from build123d import *

# Parameters (mm, degrees)
SKETCH_1_W             = 60
SKETCH_1_H             = 60
SKETCH_1_R             = 17.5
EXTRUDE_1_DEPTH        = 80
HOLE_WIZARD_M6_1_D     = 5
HOLE_WIZARD_M6_1_DEPTH = 17
HOLE_WIZARD_M6_1_TIP   = 1.502151548


with BuildPart() as part:
    # Sketch 1 → Extrude 1 (new body)
    with BuildSketch(Plane(origin=(0, 0, 0), x_dir=(0, 0, -1), z_dir=(1, 0, 0))):
        Rectangle(SKETCH_1_W, SKETCH_1_H)
        Circle(SKETCH_1_R, mode=Mode.SUBTRACT)
    extrude(amount=EXTRUDE_1_DEPTH)

    # Sketch 6 → Cut-Revolve 5 (revolve, cut)
    with BuildSketch(Plane.XY, mode=Mode.PRIVATE) as cut_revolve_5_sk:
        Polygon((0, 17.5), (2.5, 17.5), (2.5, 20.547619048), (2, 20.547619048), (2, 22.833333333), (0, 22.833333333), align=None)
    revolve(cut_revolve_5_sk.sketch.rotate(Axis((80, 0, 0), (-1, 0, 0)), 270), axis=Axis((80, 0, 0), (-1, 0, 0)), mode=Mode.SUBTRACT)

    # Sketch 7 → Cut-Revolve 6 (revolve, cut)
    with BuildSketch(Plane.XY, mode=Mode.PRIVATE) as cut_revolve_6_sk:
        Polygon((77.5, 17.5), (80, 17.5), (80, 22.833333333), (78, 22.833333333), (78, 20.547619048), (77.5, 20.547619048), align=None)
    revolve(cut_revolve_6_sk.sketch.rotate(Axis((80, 0, 0), (-1, 0, 0)), 270), axis=Axis((80, 0, 0), (-1, 0, 0)), mode=Mode.SUBTRACT)

    # Hole Wizard M6 _1
    with Locations(Plane.XY.offset(30)):
        with Locations((15, 20), (15, -20), (65, -20), (65, 20)):
            Hole(HOLE_WIZARD_M6_1_D / 2, depth=HOLE_WIZARD_M6_1_DEPTH)
            with Locations((0, 0, -(HOLE_WIZARD_M6_1_DEPTH + HOLE_WIZARD_M6_1_TIP / 2))):  # 118° drill point
                Cone(0, HOLE_WIZARD_M6_1_D / 2, HOLE_WIZARD_M6_1_TIP, mode=Mode.SUBTRACT)


solid = part.part
Can you work these out from the model? Positions are in its coordinate system, mm. A direction names the side the tool comes from. Give positions to 0.01 mm unless a question says otherwise; leave off trailing zeros. Order: outer loops, then holes, each group sorted by start corner. A loop starts at its lowest first (then second) coordinate and runs counter-clockwise, first axis right, second up. Notation, with made-up numbers: M -3.75,17.5 L 55.25,17.5 A18 cw 55.25,36.5 Z; hole C 30.25,69 d11. An arc over 180 degrees is marked long. Use one line per item in the form item = value. Start each with the question number.
Item 1: If we section it at D-D (x = 51.5): Write out the boundary of the cut face in (y, z).
Item 2: If we section it at A-A (y = 0): Write out the boundary of the cut face in (x, z), then the cut area to 3 significant figures.
Item 3: If I drill on line 1 along X through (y, z) = (20, 22); line 2 along Y through (x, z) = (15, 26); line 3 along Y through (x, z) = (55, 0), over which ranges is the centre line in solid material (lowest first)?
Item 4: If we section it at C-C (z = 25): Write out the boundary of the cut face in (x, y), then the cut area to 3 significant figures.
Item 5: Will these pins go through, and if not, where does the flat tip stop? pin 1 Ø4.5 at (x, y) = (15, -20) entering from +Z; pin 2 Ø10 at (y, z) = (-3, -15) entering from -X; pin 3 Ø4 at (x, y) = (65, 20) entering from +Z.
Item 6: For faces 1 (the cylindrical face through (16.84, -18.31, 21.38)), 2 (the flat face through (78, 9, -19)), 3 (the cylindrical face through (39.475, -10.648, 13.887)), 4 (the flat face through (2, 9, 19)), which set-ups out of +Z, -Z, +X, -X, +Y, -Y let a thin tool reach every point of the face, with its end or its side?
Item 7: We'd pull the mould along Z, two halves only. Please class faces 5 (the cylindrical face through (79, -22.3, -4.9)), 6 (the flat face through (39, 0, -30)), 7 (the flat face through (39, 30, 0)): +Z half, -Z half, draft (parallel to the pull), parting line (faces both ways), or undercut.
Outcome:
q1.outline = M -30,-30 L 30,-30 L 30,30 L -30,30 Z; hole C 0,0 d35
q2.outline = M 0,-30 L 80,-30 L 80,-22.83 L 78,-22.83 L 78,-20.55 L 77.5,-20.55 L 77.5,-17.5 L 2.5,-17.5 L 2.5,-20.55 L 2,-20.55 L 2,-22.83 L 0,-22.83 Z; M 0,22.83 L 2,22.83 L 2,20.55 L 2.5,20.55 L 2.5,17.5 L 77.5,17.5 L 77.5,20.55 L 78,20.55 L 78,22.83 L 80,22.83 L 80,30 L 0,30 Z
q2.area = 1,950 mm2
q3.line_1 = 0 to 12.5, 17.5 to 62.5, 67.5 to 80
q3.line_2 = -30 to -22.5, -17.5 to 17.5, 22.5 to 30
q3.line_3 = -30 to -17.5, 17.5 to 30
q4.outline = M 0,-30 L 80,-30 L 80,30 L 0,30 Z; hole C 15,-20 d5; hole C 15,20 d5; hole C 65,-20 d5; hole C 65,20 d5
q4.area = 4,720 mm2
q5.pin_1 = 12.85
q5.pin_2 = 2.5
q5.pin_3 = 12.7
q6.face_1 = +Z
q6.face_2 = +X
q6.face_3 = +X, -X
q6.face_4 = -X
q7.face_5 = undercut
q7.face_6 = -Z half
q7.face_7 = draft
